Work out the finished part from the listing and answer in its coordinate system (mm). Face numbers are marked on the shaded views. A direction names the side the tool comes from. Give positions to 0.01 mm unless a question says otherwise; leave off trailing zeros. Loops run counter-clockwise (first coordinate to the right, second up) from the corner with the lowest first, then second, coordinate; pieces in that order, holes last. Notation, with made-up numbers: M 55.25,24.5 L 66.25,24.5 A29 ccw 66.25,60.5 Z; hole C -23,13.5 d6. An arc over 180 degrees is marked long. Use a Markdown table: item, result.
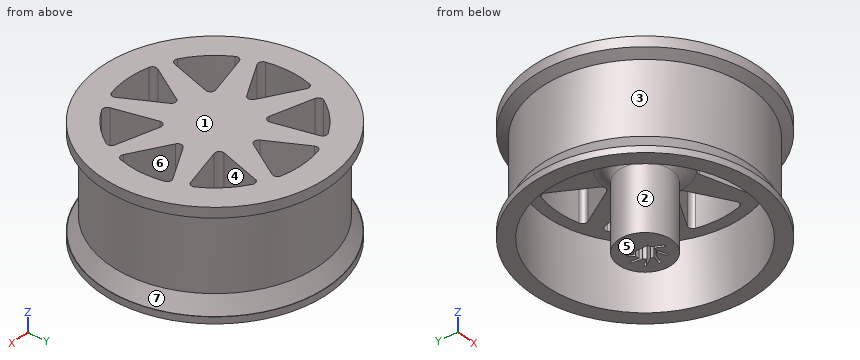
```python
from build123d import *

# Parameters (mm, degrees)
CORTAR_EXTRUIR1_REACH        = 46.176
CROQUIS3_R                   = 22.5
CROQUIS4_R                   = 22.5
CROQUIS4_R_2                 = 20
SALIENTE_EXTRUIR1_DEPTH      = 10
REDONDEO2_R                  = 1
CROQUIS6_R                   = 6
SALIENTE_EXTRUIR2_DEPTH      = 17.8
CORTAR_EXTRUIR3_DEPTH        = 9.5
CORTAR_EXTRUIR4_DEPTH        = 9.5
MATRIZC1_COUNT               = 4
MATRIZC1_ANGLE               = 120
MATRIZC1_THE_OTHER_WAY_COUNT = 4
MATRIZC1_THE_OTHER_WAY_ANGLE = 120
REDONDEO3_R                  = 3
SALIENTE_EXTRUIR3_START      = -7
SALIENTE_EXTRUIR3_DEPTH      = 7
CHAFL_N1_SIZE                = 3.464101615
CHAFL_N1_SIZE_2              = 2


with BuildPart() as part:
    # Croquis2 → Revolución2 (revolve)
    with BuildSketch(Plane(origin=(0, 0, 0), x_dir=(0, 0, -1), z_dir=(1, 0, 0)), mode=Mode.PRIVATE) as revoluci_n2_sk:
        Polygon((-10.9, 23.75), (10.9, 23.75), (10.9, 25.85), (12.4, 25.85), (12.4, 0), (-12.4, 0), (-12.4, 25.85), (-10.9, 25.85), align=None)
    revolve(revoluci_n2_sk.sketch.rotate(Axis((0, 0, 12.4), (0, 0, -1)), 90), axis=Axis((0, 0, 12.4), (0, 0, -1)))

    # Croquis3 → Cortar-Extruir1 (cut, up to next)
    with BuildSketch(Plane.XY.offset(12.4), mode=Mode.PRIVATE) as cortar_extruir1_sk1:
        Circle(CROQUIS3_R)
    cortar_extruir1_tool1 = extrude(cortar_extruir1_sk1.sketch, amount=-CORTAR_EXTRUIR1_REACH, mode=Mode.PRIVATE) & part.part
    add(cortar_extruir1_tool1.solids().sort_by_distance((0, 0, 12.4))[0], mode=Mode.SUBTRACT)

    # Croquis4 → Saliente-Extruir1 (add)
    # profile 1 of 2: a face of its own
    with BuildSketch(Plane.XY.offset(12.4)):
        Circle(CROQUIS4_R)
        Circle(CROQUIS4_R_2, mode=Mode.SUBTRACT)
    # profile 2 of 2: a face of its own
    with BuildSketch(Plane.XY.offset(12.4)):
        with BuildLine():
            Line((0, 8), (-6.270417461, 18.991626177))
            ThreePointArc((-6.270417461, 18.991626177), (-7.653668647, 18.47759065), (-8.995252948, 17.862962364))
            Line((-8.995252948, 17.862962364), (-5.656854249, 5.656854249))
            Line((-5.656854249, 5.656854249), (-17.862962364, 8.995252948))
            ThreePointArc((-17.862962364, 8.995252948), (-18.47759065, 7.653668647), (-18.991626177, 6.270417461))
            Line((-18.991626177, 6.270417461), (-8, 0))
            Line((-8, 0), (-18.991626177, -6.270417461))
            ThreePointArc((-18.991626177, -6.270417461), (-18.47759065, -7.653668647), (-17.862962364, -8.995252948))
            Line((-17.862962364, -8.995252948), (-5.656854249, -5.656854249))
            Line((-5.656854249, -5.656854249), (-8.995252948, -17.862962364))
            ThreePointArc((-8.995252948, -17.862962364), (-7.653668647, -18.47759065), (-6.270417461, -18.991626177))
            Line((-6.270417461, -18.991626177), (0, -8))
            Line((0, -8), (6.270417461, -18.991626177))
            ThreePointArc((6.270417461, -18.991626177), (7.653668647, -18.47759065), (8.995252948, -17.862962364))
            Line((8.995252948, -17.862962364), (5.656854249, -5.656854249))
            Line((5.656854249, -5.656854249), (17.862962364, -8.995252948))
            ThreePointArc((17.862962364, -8.995252948), (18.47759065, -7.653668647), (18.991626177, -6.270417461))
            Line((18.991626177, -6.270417461), (8, 0))
            Line((8, 0), (18.991626177, 6.270417461))
            ThreePointArc((18.991626177, 6.270417461), (18.47759065, 7.653668647), (17.862962364, 8.995252948))
            Line((17.862962364, 8.995252948), (5.656854249, 5.656854249))
            Line((5.656854249, 5.656854249), (8.995252948, 17.862962364))
            ThreePointArc((8.995252948, 17.862962364), (7.653668647, 18.47759065), (6.270417461, 18.991626177))
            Line((6.270417461, 18.991626177), (0, 8))
        make_face()
    extrude(amount=-SALIENTE_EXTRUIR1_DEPTH)

    # Redondeo2
    redondeo2_edges = [part.edges().sort_by_distance(p)[0] for p in [
        (18.991626177, -6.270417461, 7.4),
        (18.991626177, 6.270417461, 7.4),
        (8.995252948, -17.862962364, 7.4),
        (17.862962364, -8.995252948, 7.4),
        (-6.270417461, -18.991626177, 7.4),
        (6.270417461, -18.991626177, 7.4),
        (-17.862962364, -8.995252948, 7.4),
        (-8.995252948, -17.862962364, 7.4),
        (-18.991626177, 6.270417461, 7.4),
        (-18.991626177, -6.270417461, 7.4),
        (-8.995252948, 17.862962364, 7.4),
        (-17.862962364, 8.995252948, 7.4),
        (6.270417461, 18.991626177, 7.4),
        (-6.270417461, 18.991626177, 7.4),
        (17.862962364, 8.995252948, 7.4),
        (8.995252948, 17.862962364, 7.4),
        (8, 0, 7.4),
        (5.656854249, -5.656854249, 7.4),
        (0, -8, 7.4),
        (-5.656854249, -5.656854249, 7.4),
        (-8, 0, 7.4),
        (-5.656854249, 5.656854249, 7.4),
        (0, 8, 7.4),
        (5.656854249, 5.656854249, 7.4),
    ]]
    fillet(redondeo2_edges, radius=REDONDEO2_R)

    # Croquis6 → Saliente-Extruir2 (add)
    with BuildSketch(Plane(origin=(0, 0, 2.4), x_dir=(-1, 0, 0), z_dir=(0, 0, -1))):
        with Locations(Location((0, 0, 0), (0, 0, 180))):
            Circle(CROQUIS6_R)
    extrude(amount=SALIENTE_EXTRUIR2_DEPTH)

    # Croquis7 → Cortar-Extruir3 (cut)
    with BuildSketch(Plane(origin=(0, 0, -15.4), x_dir=(-1, 0, 0), z_dir=(0, 0, -1))):
        with BuildLine():
            Line((1.35, -1.542724862), (1.35, 1.542724862))
            ThreePointArc((1.35, 1.542724862), (-2.05, 0), (1.35, -1.542724862))
        make_face()
    extrude(amount=-CORTAR_EXTRUIR3_DEPTH, mode=Mode.SUBTRACT)

    # Croquis8 → Cortar-Extruir4 (cut)
    with BuildSketch(Plane(origin=(0, 0, -15.4), x_dir=(-1, 0, 0), z_dir=(0, 0, -1))):
        with BuildLine():
            Line((-1.837063356, -0.909779217), (-3.938686891, -0.238134803))
            ThreePointArc((-3.938686891, -0.238134803), (-4.100717717, 0.076103978), (-3.786478936, 0.238134803))
            Line((-3.786478936, 0.238134803), (-2.024056773, -0.325106415))
            ThreePointArc((-2.024056773, -0.325106415), (-1.995828785, -0.468153243), (-1.957504486, -0.608831821))
            ThreePointArc((-1.957504486, -0.608831821), (-1.903241606, -0.761689824), (-1.837063356, -0.909779217))
        make_face()
    cortar_extruir4 = extrude(amount=-CORTAR_EXTRUIR4_DEPTH, mode=Mode.SUBTRACT)

    # MatrizC1: Cortar-Extruir4 ×4 about axis
    matrizc1_axis = Axis((0, 0, 0), (0, 0, -1))
    for i in range(1, MATRIZC1_COUNT):
        add(cortar_extruir4.rotate(matrizc1_axis, i * MATRIZC1_ANGLE / (MATRIZC1_COUNT - 1)), mode=Mode.SUBTRACT)

    # MatrizC1 the other way: Cortar-Extruir4 ×4 about axis
    matrizc1_the_other_way_axis = Axis((0, 0, 0), (0, 0, 1))
    for i in range(1, MATRIZC1_THE_OTHER_WAY_COUNT):
        add(cortar_extruir4.rotate(matrizc1_the_other_way_axis, i * MATRIZC1_THE_OTHER_WAY_ANGLE / (MATRIZC1_THE_OTHER_WAY_COUNT - 1)), mode=Mode.SUBTRACT)

    # Redondeo3
    redondeo3_edges = [part.edges().sort_by_distance(p)[0] for p in [
        (-6, 0, 2.4),
    ]]
    fillet(redondeo3_edges, radius=REDONDEO3_R)

    # Croquis9 → Saliente-Extruir3 (add)
    with BuildSketch(Plane(origin=(0, 0, -15.4), x_dir=(-1, 0, 0), z_dir=(0, 0, -1)).offset(SALIENTE_EXTRUIR3_START)):
        with BuildLine():
            Line((1.35, 1.542724862), (1.35, -1.542724862))
            Line((1.35, -1.542724862), (1.35, -5.846152581))
            ThreePointArc((1.35, -5.846152581), (6, 0), (1.35, 5.846152581))
            Line((1.35, 5.846152581), (1.35, 1.542724862))
        make_face()
    extrude(amount=SALIENTE_EXTRUIR3_DEPTH)

    # Chaflán1
    # the kernel refuses this chamfer: 3.464101615, 2 mm, written as the material it adds along each edge
    with BuildSketch(Plane(origin=(0, 0, -10.9), x_dir=(1, 0, 0), z_dir=(0, 1, 0))) as chafl_n1_piece_1:
        Polygon((23.75, -CHAFL_N1_SIZE), (23.75 + CHAFL_N1_SIZE_2, 0), (23.75, 0), align=None)
    revolve(axis=Axis((0, 0, -10.9), (0, 0, -1)))
    with BuildSketch(Plane(origin=(0, 0, 10.9), x_dir=(1, 0, 0), z_dir=(0, 1, 0))) as chafl_n1_piece_2_section:
        Polygon((23.75 + CHAFL_N1_SIZE, 0), (23.75, CHAFL_N1_SIZE_2), (23.75, 0), align=None)
    chafl_n1_piece_2 = revolve(axis=Axis((0, 0, 10.9), (0, 0, -1)), mode=Mode.PRIVATE)
    chafl_n1_piece_2 = chafl_n1_piece_2 & Plane(origin=(0, 0, 9.540393741), x_dir=(1, 0, 0), z_dir=(0, 0, -1)) * Cylinder(25.85, 109, mode=Mode.PRIVATE)
    add(chafl_n1_piece_2)


solid = part.part
```
(1) Consider probe 1 along Y at (x, z) = (0, -2.5); probe 2 along Y at (x, z) = (-15, 6); probe 3 along X at (y, z) = (-4, 10.75). Determine where each line is inside the solid, lowest interval first. Write a range as [from, to].
Entries:
| item | result |
|---|---|
| probe 1 | y = [-23.75, -22.5], [-6, 6], [22.5, 23.75] |
| probe 2 | y = [-18.41, -13.23], [-8.21, -3.99], [3.99, 8.21], [13.23, 18.41] |
| probe 3 | x = [-25.54, -19.6], [-15.01, 15.01], [19.6, 25.54] |
(2) A cutting plane is placed at A-A (z = -9.75). Count the separate pieces of the cut face and the enclosed holes in it, and give its area (3 significant figures).
Entries:
| item | result |
|---|---|
| separate pieces | 2 |
| enclosed holes | 2 |
| area | 482 mm² |
(3) The mould has two halves that part along X. Classify the marked faces 5, 6 and 7: released by +X, released by -X, zero draft, split by the parting line, or undercut.
Entries:
| item | result |
|---|---|
| face 5 | zero draft |
| face 6 | undercut |
| face 7 | split by the parting line |
(4) A cutting plane is placed at B-B (z = -2.75). Write down the section's boundary in (x, y).
Entries:
| item | result |
|---|---|
| outline | C 0,0 d47.5; C 0,0 d12; hole C 0,0 d45 |
(5) Which of the six approach directions +Z, -Z, +X, -X, +Y, -Y give full straight-line access (tool end or side, diameter ignored) to the marked faces 1, 2, 3 and 4?
Entries:
| item | result |
|---|---|
| face 1 | +Z, +X, -X, +Y, -Y |
| face 2 | -Z |
| face 3 | none |
| face 4 | +Z, -Z |
(6) Given P1, Ø0.5, axis at y = 2.5, z = -12.5, coming from the +X side; P2, Ø10, axis at y = 13, z = -11.5, coming from the -X side; P3, Ø2, axis at y = -6.5, z = 3, coming from the +X side, each flat-ended and moving along its own axis, determine where each tip first touches the part or whether it passes through.
Entries:
| item | result |
|---|---|
| P1 | stops at x = 25.75 |
| P2 | stops at x = -24.58 |
| P3 | stops at x = 23.1 |
